Geometry check sheet. Reference: the model listing, model coordinates, mm. A direction names the side the tool comes from. Give positions to 0.01 mm unless a question says otherwise; leave off trailing zeros. Order: outer loops, then holes, each group sorted by start corner. A loop starts at its lowest first (then second) coordinate and runs counter-clockwise, first axis right, second up. Notation, with made-up numbers: M -38,-39.75 L 0,-39.75 A17 ccw 0,-22.75 Z; hole C 10.5,-36 d4. An arc over 180 degrees is marked long. Answer as CSV lines item,"result".
from build123d import *

# Parameters (mm, degrees)
SKETCH1_R           = 4.6
SKETCH1_R_2         = 3.6
BOSS_EXTRUDE1_DEPTH = 4
BOSS_EXTRUDE2_START = -4
SKETCH2_R           = 7.5
SKETCH2_R_2         = 4.6
BOSS_EXTRUDE2_DEPTH = 4
FILLET1_R           = 5


with BuildPart() as part:
    # Sketch1 → Boss-Extrude1 (new body)
    with BuildSketch(Plane(origin=(0, 0, 0), x_dir=(1, 0, 0), z_dir=(0, 1, 0))):
        with BuildLine():
            Line((6, 0), (6, -26.5))
            ThreePointArc((6, -26.5), (0, -32.5), (-6, -26.5))
            Line((-6, -26.5), (-6, 0))
            ThreePointArc((-6, 0), (0, 6), (6, 0))
        make_face()
        with Locations(Location((0, 0, 0), (0, 0, 270))):
            Circle(SKETCH1_R, mode=Mode.SUBTRACT)
        with Locations(Location((0, -26.5, 0), (0, 0, 270))):
            Circle(SKETCH1_R_2, mode=Mode.SUBTRACT)
    extrude(amount=BOSS_EXTRUDE1_DEPTH)

    # Sketch2 → Boss-Extrude2 (add)
    with BuildSketch(Plane(origin=(0, 4, 0), x_dir=(1, 0, 0), z_dir=(0, 1, 0)).offset(BOSS_EXTRUDE2_START)):
        Circle(SKETCH2_R)
        with Locations(Location((0, 0, 0), (0, 0, 270))):
            Circle(SKETCH2_R_2, mode=Mode.SUBTRACT)
    extrude(amount=BOSS_EXTRUDE2_DEPTH)

    # Fillet1
    fillet1_edges = [part.edges().sort_by_distance(p)[0] for p in [
        (6, 2, 4.5),
        (-6, 2, 4.5),
    ]]
    fillet(fillet1_edges, radius=FILLET1_R)

    # Chamfer2
    # the kernel refuses this chamfer: 1 mm, written as the material it takes off along each edge
    with BuildSketch(Plane(origin=(0, 4, 0), x_dir=(-0.8800000000000001, 0, 0.47497368348151653), z_dir=(0.47497368348151653, 0, 0.8800000000000001))) as chamfer2_piece_1:
        with BuildLine():
            Line((6.471715729, -0.028284271), (7.528284271, 1.028284271))
            Line((7.528284271, 1.028284271), (7.548284271, 1.028284271))
            ThreePointArc((7.548284271, 1.028284271), (7.52, 0.514142136), (7.52, 0))
            Line((7.52, 0), (7.5, -0.02))
            ThreePointArc((7.5, -0.02), (6.985857864, -0.02), (6.471715729, -0.048284271))
            Line((6.471715729, -0.048284271), (6.471715729, -0.028284271))
        make_face()
    revolve(axis=Axis((0, 4, 0), (0, -1, 0)), revolution_arc=236.715273153, mode=Mode.SUBTRACT)
    with BuildSketch(Plane(origin=(11, 4, 5.937171044), x_dir=(-0.33003370038362406, 0, 0.9439691502433181), z_dir=(0.9439691502433181, 0, 0.33003370038362406))) as chamfer2_piece_2:
        with BuildLine():
            Line((6.028284271, -0.028284271), (4.971715729, 1.028284271))
            Line((4.971715729, 1.028284271), (4.951715729, 1.028284271))
            ThreePointArc((4.951715729, 1.028284271), (4.98, 0.514142136), (4.98, 0))
            Line((4.98, 0), (5, -0.02))
            ThreePointArc((5, -0.02), (5.514142136, -0.02), (6.028284271, -0.048284271))
            Line((6.028284271, -0.048284271), (6.028284271, -0.028284271))
        make_face()
    revolve(axis=Axis((11, 4, 5.937171044), (0, -1, 0)), revolution_arc=99.086815597, mode=Mode.SUBTRACT)
    with BuildSketch(Plane(origin=(-11, 4, 5.937171044), x_dir=(0.3300337003836236, 0, 0.9439691502433183), z_dir=(-0.9439691502433183, 0, 0.3300337003836236))) as chamfer2_piece_3:
        with BuildLine():
            Line((4.971715729, -1.028284271), (6.028284271, 0.028284271))
            Line((6.028284271, 0.028284271), (6.028284271, 0.048284271))
            ThreePointArc((6.028284271, 0.048284271), (5.514142136, 0.02), (5, 0.02))
            Line((5, 0.02), (4.98, 0))
            ThreePointArc((4.98, 0), (4.98, -0.514142136), (4.951715729, -1.028284271))
            Line((4.951715729, -1.028284271), (4.971715729, -1.028284271))
        make_face()
    revolve(axis=Axis((-11, 4, 5.937171044), (0, 1, 0)), revolution_arc=99.086815597, mode=Mode.SUBTRACT)


solid = part.part
(1) Section check B-B on x = 0. Enter the section's corners in (y, z).
The answers:
outline,"M 0,-7.5 L 3,-7.5 L 4,-6.5 L 4,-4.6 L 0,-4.6 Z; M 0,4.6 L 4,4.6 L 4,22.9 L 0,22.9 Z; M 0,30.1 L 4,30.1 L 4,32.5 L 0,32.5 Z"
(2) Section check C-C on y = 2. Enter the section's corners in (x, z), then the cut area to 3 significant figures.
The answers:
outline,"M -6.6,3.56 A7.5 ccw long 6.6,3.56 A5 cw 6,5.94 L 6,26.5 A6 ccw -6,26.5 L -6,5.94 A5 cw Z; hole C 0,0 d9.2; hole C 0,26.5 d7.2"
area,"365 mm2"
(3) Draft check along Z on faces 3 (the face through (-6, 2, 16)), 4 (the face through (1.38, 1.97, 4.39)), 5 (the face through (-6.157, 1.479, 4.696)), 6 (the face through (0.158, 1.972, 22.903)). Enter one of: +Z half, -Z half, draft (parallel to the pull), parting line (faces both ways), or undercut.
The answers:
face 3,"draft"
face 4,"undercut"
face 5,"+Z half"
face 6,"undercut"
(4) Section check D-D on z = 28. Enter the section's corners in (x, y).
The answers:
outline,"M -5.81,0 L -3.27,0 L -3.27,4 L -5.81,4 Z; M 3.27,0 L 5.81,0 L 5.81,4 L 3.27,4 Z"
(5) Material ranges on line 1 (X direction, y = 3.1, z = 26.5); line 2 (Z direction, x = -1, y = 3.4); line 3 (Z direction, x = -1, y = 2.05), recorded low to high.
The answers:
line 1,"x = -6 to -3.6, 3.6 to 6"
line 2,"z = -7.03 to -4.49, 4.49 to 23.04, 29.96 to 32.42"
line 3,"z = -7.43 to -4.49, 4.49 to 23.04, 29.96 to 32.42"
(6) Tool access check on faces 1 (the face through (0, 4, 13)), 2 (the face through (6, 2, 16)). Record the directions out of +Z, -Z, +X, -X, +Y, -Y that give a thin tool (end or side, any length) a straight path to the whole face; none if there is none.
The answers:
face 1,"+Z, -Z, +X, -X, +Y"
face 2,"+Z, +X, +Y, -Y"
(7) Section check A-A on z = 0. Enter the section's corners in (x, y), then the cut area to 3 significant figures.
The answers:
outline,"M -7.5,0 L -4.6,0 L -4.6,4 L -6.5,4 L -7.5,3 Z; M 4.6,0 L 7.5,0 L 7.5,3 L 6.5,4 L 4.6,4 Z"
area,"22.2 mm2"
(8) Gauge pin test, flat ends, axial feed: P1, Ø1.5, axis at x = -4.5, y = 1.5, coming from the -Z side; P2, Ø2, axis at y = 2, z = 16, coming from the -X side. Record the tip position at first contact, or that the pin passes through.
The answers:
P1,"stops at z = -6.5"
P2,"stops at x = -6"
